Part model, mm, in its own coordinate system. Face numbers are marked on the shaded views. A direction names the side the tool comes from. Round coordinates to 2 decimals unless told otherwise and drop trailing zeros. Order: outer loops, then holes, each group sorted by start corner. A loop starts at its lowest first (then second) coordinate and runs counter-clockwise, first axis right, second up. Notation, with made-up numbers: M 27.5,26 L 38.5,26 A21 ccw 38.5,64 Z; hole C 86,70.25 d8. An arc over 180 degrees is marked long. One line per question, with ' | ' between items.
from build123d import *

# Parameters (mm, degrees)
CYLINDER017_R         = 1.9
CYLINDER017_DEPTH     = 5
CYLINDER016_R         = 1.6
CYLINDER016_DEPTH     = 30.25
CYLINDER013_R         = 3.75
CYLINDER013_DEPTH     = 7.25
BOX028_W              = 6
BOX028_H              = 16
BOX028_DEPTH          = 7.5
CHAMFER006006014_SIZE = 3
CYLINDER015_R         = 8
CYLINDER015_DEPTH     = 6
CHAMFER006006017_SIZE = 3
BOX029_W              = 3
BOX029_H              = 6
BOX029_DEPTH          = 6
CYLINDER014_R         = 3.75
CYLINDER014_DEPTH     = 7.25
CHAMFER006006018_SIZE = 0.4
CHAMFER006006020_SIZE = 1


with BuildPart() as cylinder017:
    # Cylinder017 → Cylinder017 (new body)
    with BuildSketch(Plane(origin=(8.25, 15, 22), x_dir=(0, 0, 1), z_dir=(-1, 0, 0))):
        Circle(CYLINDER017_R)
    extrude(amount=CYLINDER017_DEPTH)


with BuildPart() as fusion008:
    # Cylinder016 → Cylinder016 (new body)
    with BuildSketch(Plane(origin=(9.25, 15, 22), x_dir=(0, 0, 1), z_dir=(-1, 0, 0))):
        Circle(CYLINDER016_R)
    extrude(amount=CYLINDER016_DEPTH)

    # Fusion008: union Cylinder017
    add(cylinder017.part)


with BuildPart() as fusion008_1:
    # Fusion008 placement: moved
    add(fusion008.part.moved(Location((-0.25, 0, 0))))


with BuildPart() as cylinder013:
    # Cylinder013 → Cylinder013 (new body)
    with BuildSketch(Plane(origin=(2.25, 15, 22), x_dir=(0, 0, 1), z_dir=(-1, 0, 0))):
        Circle(CYLINDER013_R)
    extrude(amount=CYLINDER013_DEPTH)


with BuildPart() as chamfer006006014:
    # Box028 → Box028 (new body)
    with BuildSketch(Plane(origin=(2, 7, 18.25), x_dir=(1, 0, 0), z_dir=(0, 0, 1))):
        with Locations((3, 8)):
            Rectangle(BOX028_W, BOX028_H)
    extrude(amount=BOX028_DEPTH)

    # Chamfer006006014
    chamfer006006014_edges = [chamfer006006014.edges().sort_by_distance(p)[0] for p in [
        (8, 7, 22),
        (8, 23, 22),
    ]]
    chamfer(chamfer006006014_edges, length=CHAMFER006006014_SIZE)


with BuildPart() as chamfer006006014_1:
    # Chamfer006006014 placement: moved
    add(chamfer006006014.part.moved(Location((0.25, 0, 0))))


with BuildPart() as common003:
    # Cylinder015 → Cylinder015 (new body)
    with BuildSketch(Plane(origin=(2.25, 15, 22), x_dir=(0, 0, -1), z_dir=(1, 0, 0))):
        Circle(CYLINDER015_R)
    extrude(amount=CYLINDER015_DEPTH)

    # Chamfer006006017
    chamfer006006017_edges = [common003.edges().sort_by_distance(p)[0] for p in [
        (8.25, 15, 30),
    ]]
    chamfer(chamfer006006017_edges, length=CHAMFER006006017_SIZE)

    # Common003: intersect Chamfer006006014
    add(chamfer006006014_1.part, mode=Mode.INTERSECT)


with BuildPart() as common003_1:
    # Common003 placement: moved
    add(common003.part.moved(Location((-0.25, 0, 0))))


with BuildPart() as cube028:
    # Box029 → Box029 (new body)
    with BuildSketch(Plane(origin=(-8, 12, 19), x_dir=(1, 0, 0), z_dir=(0, 0, 1))):
        with Locations((1.5, 3)):
            Rectangle(BOX029_W, BOX029_H)
    extrude(amount=BOX029_DEPTH)


with BuildPart() as chamfer006006020:
    # Cylinder014 → Cylinder014 (new body)
    with BuildSketch(Plane(origin=(-3.75, 15, 22), x_dir=(0, 0, 1), z_dir=(-1, 0, 0))):
        Circle(CYLINDER014_R)
    extrude(amount=CYLINDER014_DEPTH)

    # Common: intersect Cube028
    add(cube028.part, mode=Mode.INTERSECT)

    # Fusion011: union Cylinder013, Common003
    add(cylinder013.part)
    add(common003_1.part)

    # Cut002004005002: cut Fusion008
    add(fusion008_1.part, mode=Mode.SUBTRACT)

    # Chamfer006006018
    chamfer006006018_edges = [chamfer006006020.edges().sort_by_distance(p)[0] for p in [
        (8, 15, 20.1),
    ]]
    chamfer(chamfer006006018_edges, length=CHAMFER006006018_SIZE)

    # Chamfer006006020
    chamfer006006020_edges = [chamfer006006020.edges().sort_by_distance(p)[0] for p in [
        (2, 22.763156, 20.067796),
        (2, 22.763156, 23.932204),
        (2, 7.236844, 20.067796),
        (2, 7.236844, 23.932204),
    ]]
    chamfer(chamfer006006020_edges, length=CHAMFER006006020_SIZE)


solid = chamfer006006020.part
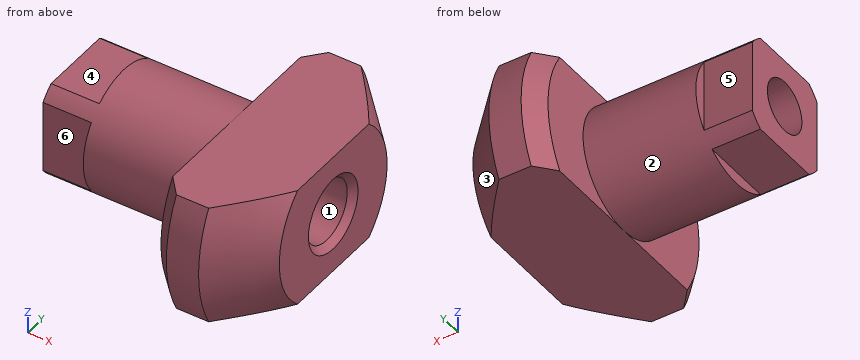
1) Saw through at D-D (x = 6.75). List the corners of the cut face in (y, z), plus the area to 3 significant figures.
The answers:
outline: M 10,18.25 L 20,18.25 A6.25 ccw 20,25.75 L 10,25.75 A6.25 ccw Z; hole C 15,22 d3.8 | area: 76.4 mm²
2) Drop flat-ended pins along their axis: pin 1 (3.5 mm diameter, centred on x = -6, z = 22.5, fed in from +Y); pin 2 (1.5 mm diameter, centred on y = 15.5, z = 21.5, fed in from -X); pin 3 (0.6 mm diameter, centred on y = 14, z = 25.5, fed in from -X); pin 4 (1.5 mm diameter, centred on x = -7, y = 15.5, fed in from -Z). Give the stop position or say it passes through.
The answers:
pin 1: stops at y = 18.75 | pin 2: passes through | pin 3: stops at x = -5 | pin 4: stops at z = 19
3) Saw through at B-B (x = -6.5). List the corners of the cut face in (y, z), plus the area to 3 significant figures.
The answers:
outline: M 12,19.75 A3.75 ccw 12.75,19 L 17.25,19 A3.75 ccw 18,19.75 L 18,24.25 A3.75 ccw 17.25,25 L 12.75,25 A3.75 ccw 12,24.25 Z; hole C 15,22 d3.2 | area: 26.9 mm²
4) Two-plate mould, pull along Y, no slides. Class the marked faces 1, 2 and 3: released by +Y, released by -Y, zero draft, split by the parting line, or undercut.
The answers:
face 1: undercut | face 2: split by the parting line | face 3: released by +Y
5) Which spindle directions (+Z, -Z, +X, -X, +Y, -Y) get a long thin tool onto all of the face, cutting with end or side? Do the marked faces 4, 5 and 6. Say none if no direction does.
The answers:
face 4: +Z, -X, +Y, -Y | face 5: +Z, -Z, -X, +Y | face 6: +Z, -Z, -X, -Y
6) Probe line 1 (Z direction, x = -2, y = 15); line 2 (Y direction, x = -0.75, z = 22); line 3 (Y direction, x = 4.85, z = 22). List the from-to ranges inside material, lowest first. Write a range as [from, to].
The answers:
line 1: z = [18.25, 20.4], [23.6, 25.75] | line 2: y = [11.25, 13.4], [16.6, 18.75] | line 3: y = [7, 13.1], [16.9, 23]
7) Saw through at C-C (y = 12.25). List the corners of the cut face in (x, z).
The answers:
outline: M -8,19.45 L 2,19.45 L 2,18.25 L 8,18.25 L 8,25.75 L 2,25.75 L 2,24.55 L -8,24.55 Z
8) Saw through at A-A (z = 22). List the corners of the cut face in (x, y).
The answers:
outline: M -8,12 L -5,12 L -5,11.25 L 2,11.25 L 2,8 L 3,7 L 5,7 L 8,10 L 8,12.7 L 7.6,13.1 L 3,13.1 L 3,13.4 L -8,13.4 Z; M -8,16.6 L 3,16.6 L 3,16.9 L 7.6,16.9 L 8,17.3 L 8,20 L 5,23 L 3,23 L 2,22 L 2,18.75 L -5,18.75 L -5,18 L -8,18 Z
